Geometry check sheet. Reference: the model listing, model coordinates, mm. Give positions to 0.01 mm unless a question says otherwise; leave off trailing zeros. Write each loop counter-clockwise with the first axis right and the second up, starting at its lowest first coordinate (ties: lowest second). Pieces come first, ordered by that corner, then holes. Notation, with made-up numbers: (34.5, -36.75) -> (67.5, -36.75) arc R21 cw to (67.5, -2.75) -> close; hole circle Ø6 at (7, -4). An arc over 180 degrees is marked (long way). Write item = value, one per line. Start each with the question number.
1. Depth check by flat-ended pin: P1, Ø5, axis at y = -3.5, z = 3, coming from the -X side. Enter the tip coordinate at first touch or a pass-through.
2. Thickness scan on line 1 along Z through (x, y) = (-66.5, -4); line 2 along Z through (x, y) = (80.5, -3.25); line 3 along X through (y, z) = (-2.75, 7). Record the ranges inside material, lowest first.
3. Cross-section at A-A, the plane x = -61.5. Record the cut outline in (y, z).
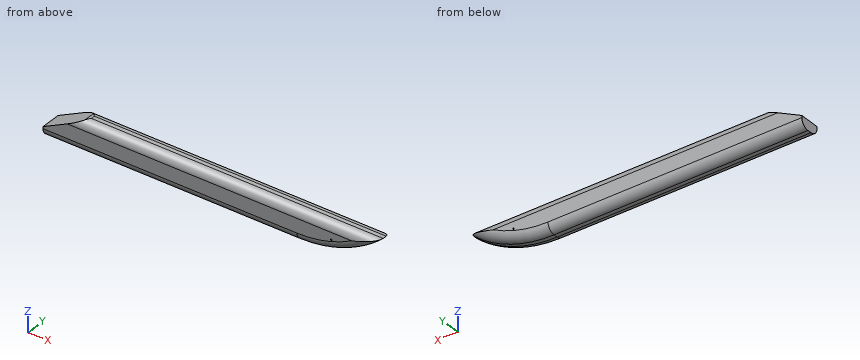
```python
from build123d import *

# Parameters (mm, degrees)
F0_W        = 209.9508528371
F0_H        = 19.0544301776
F0_R        = 0.4554012186
F1_DEPTH    = 12.7
F2_T1_DEPTH = 264.7329269001
F3_SIZE2    = 25.4
F3_SIZE     = 12.7
F4_R        = 5.08


# Not quite as in the source:
# - a fillet or chamfer that OpenCascade refuses, or shapes differently, is made with other operations: its cross-section is extruded or revolved along the edge and cut away or added


with BuildPart() as f1:
    # F0 (on Front) → F1 (new body)
    with BuildSketch(Plane.XZ):
        Rectangle(F0_W, F0_H)
        with Locations((76.2023702264, 0)):
            Circle(F0_R, mode=Mode.SUBTRACT)
    extrude(amount=F1_DEPTH)

    # F2: fillet of radius 76.2 on 1 edges, made by hand

    # F2_s2 → F2_t1 (cut)
    with BuildSketch(Plane.XZ.offset(-126.0164634501)):
        with BuildLine():
            ThreePointArc((54.5688410385, -9.5272150888), (81.5127418283, -4.6046042822), (104.9754264186, 9.5272150888))
            Line((104.9754264186, 9.5272150888), (104.9754264186, -9.5272150888))
            Line((104.9754264186, -9.5272150888), (54.5688410385, -9.5272150888))
        make_face()
    extrude(amount=F2_T1_DEPTH, mode=Mode.SUBTRACT)

    # F3
    f3_edges = [f1.edges().sort_by_distance(p)[0] for p in [
        (-104.975426, -6.35, 9.527215),
    ]]
    f3_side = f1.faces().sort_by_distance((-104.975426, -6.35, 0))[0]
    chamfer(f3_edges, length=F3_SIZE, length2=F3_SIZE2, reference=f3_side)

    # F4
    f4_edges = [f1.edges().sort_by_distance(p)[0] for p in [
        (81.512742, -12.7, -4.604604),
        (12.7, -12.7, 9.527215),
        (12.7, 0, 9.527215),
        (-25.203293, 0, -9.527215),
        (-79.575426, -6.35, 9.527215),
        (-25.203293, -12.7, -9.527215),
        (81.512742, 0, -4.604604),
    ]]
    fillet(f4_edges, radius=F4_R)


solid = f1.part
```
Answers:
q1.P1 = -97.63
q2.line_1 = -9.41 to 9.41
q2.line_2 = -4.62 to 9.19
q2.line_3 = -84.63 to 101.04
q3.outline = (-12.7, -4.45) arc R5.08 ccw to (-7.62, -9.53) -> (-5.08, -9.53) arc R5.08 ccw to (0, -4.45) -> (0, 4.45) arc R5.08 ccw to (-5.08, 9.53) -> (-7.62, 9.53) arc R5.08 ccw to (-12.7, 4.45) -> close
